Verification items for the finished model (mm, model axes). A direction names the side the tool comes from. Round coordinates to 2 decimals unless told otherwise and drop trailing zeros. Order: outer loops, then holes, each group sorted by start corner. A loop starts at its lowest first (then second) coordinate and runs counter-clockwise, first axis right, second up. Notation, with made-up numbers: (76, 79) -> (106, 79) arc R24 cw to (106, 116) -> close; hole circle Ø6 at (65.25, 62.25). An arc over 180 degrees is marked (long way). Return JSON: item names as keys, results as strings. Group by question number.
Item 1: Sectioned sample at A-A on x = 0. Record the cut outline in (y, z), plus the area to 3 significant figures.
Item 2: Depth check by flat-ended pin: pin 1 Ø9.5 at (x, y) = (-31.75, 54.99) entering from +Z; pin 2 Ø4 at (y, z) = (23, 4) entering from -X; pin 3 Ø5 at (y, z) = (31, 6) entering from -X. Enter the tip coordinate at first touch or a pass-through.
Item 3: Sectioned sample at B-B on z = -3.5. Record the cut outline in (x, y), plus the area to 3 significant figures.
Item 4: Access from +Z, -Z, +X, -X, +Y, -Y to the whole of each face (thin tool, end or side, straight path). Record for faces 4 (the cylindrical face through (-33.4, 51.83, 4.46)), 5 (the flat face through (62, 12.7, -3)).
Item 5: Scan lines: probe 1 along X at (y, z) = (31.75, 6.5); probe 2 along X at (y, z) = (67.5, 4.75); probe 3 along Z at (x, y) = (-49, 44). Record each from-to range of solid material in increasing order. Write a range as from..to.
Item 6: Draft check along X on faces 1 (the flat face through (-53, 2, 0)), 2 (the cylindrical face through (-58.29, 30.38, 4.46)), 3 (the flat face through (-1, 56, 12.7)). Enter one of: pulls with the +X half, pulls with the -X half, needs draft (parallel to the pull), parting line crosses it, or undercut.
Item 7: Sectioned sample at C-C on y = 42. Record the cut outline in (x, z), plus the area to 3 significant figures.
Item 8: Sectioned sample at D-D on z = 5. Record the cut outline in (x, y), plus the area to 3 significant figures.
```python
from build123d import *

# Parameters (mm, degrees)
F1_DEPTH       = 12.7
F3_DEPTH       = 6.35
F5_D           = 7.1374
F5_CSINK_D     = 13.4874
F5_CSINK_ANGLE = 82


with BuildPart() as f1:
    # F0 (on Top) → F1 (new body)
    with BuildSketch(Plane.XY):
        with BuildLine():
            Line((-76.2, 0), (-50.8, 0))
            ThreePointArc((-50.8, 0), (0, 50.8), (50.8, 0))
            Line((50.8, 0), (76.2, 0))
            ThreePointArc((76.2, 0), (0, 76.2), (-76.2, 0))
        make_face()
    extrude(amount=F1_DEPTH)

    # F2 (on face) → F3 (join)
    with BuildSketch(Plane(origin=(0, 0, 0), x_dir=(1, 0, 0), z_dir=(0, 0, -1))):
        with BuildLine():
            Line((-74.9170394667, -12.7), (-49.5170394667, -12.7))
            ThreePointArc((-49.5170394667, -12.7), (-49.581350313, -11.4235362865), (-49.7736315316, -10.1600002047))
            ThreePointArc((-49.7736315316, -10.1600002047), (-54.1848541289, -2.8626223667), (-62.2170394667, 0))
            ThreePointArc((-62.2170394667, 0), (-71.1972955878, -3.7197438789), (-74.9170394667, -12.7))
        make_face()
        with BuildLine():
            ThreePointArc((62.2170394667, 0), (54.1848541308, -2.8626223652), (49.7736315325, -10.1600001999))
            ThreePointArc((49.7736315325, -10.1600001999), (49.5813503133, -11.423536284), (49.5170394667, -12.7))
            Line((49.5170394667, -12.7), (74.9170394667, -12.7))
            ThreePointArc((74.9170394667, -12.7), (71.1972955878, -3.7197438789), (62.2170394667, 0))
        make_face()
    extrude(amount=F3_DEPTH)

    # F5 (through all)
    with Locations(Plane.XY.offset(12.7)):
        with Locations((-54.9926131403, 31.75), (-31.75, 54.9926131403), (0, 63.5), (31.75, 54.9926131403), (54.9926131403, 31.75)):
            CounterSinkHole(F5_D / 2, F5_CSINK_D / 2, counter_sink_angle=F5_CSINK_ANGLE)


solid = f1.part
```
Recorded:
{
 "1": {"outline": "(50.8, 0) -> (59.93, 0) -> (59.93, 9.05) -> (56.76, 12.7) -> (50.8, 12.7) -> close; (67.07, 0) -> (76.2, 0) -> (76.2, 12.7) -> (70.24, 12.7) -> (67.07, 9.05) -> close", "area": "220 mm²"},
 "2": {"pin 1": "z = 10.41", "pin 2": "x = -73.25", "pin 3": "x = -70.67"},
 "3": {"outline": "(-74.92, 12.7) arc R12.7 ccw to (-49.52, 12.7) -> close; (49.52, 12.7) arc R12.7 ccw to (74.92, 12.7) -> close", "area": "507 mm²"},
 "4": {"face 4": "+Z, -Z", "face 5": "-Z, +X, -X, +Y"},
 "5": {"probe 1": "-69.27..-58.56, -51.42..-39.66, 39.66..51.42, 58.56..69.27", "probe 2": "-35.36..35.36", "probe 3": "0..12.7"},
 "6": {"face 1": "undercut", "face 2": "undercut", "face 3": "needs draft"},
 "7": {"outline": "(-63.58, 0) -> (-28.58, 0) -> (-28.58, 12.7) -> (-63.58, 12.7) -> close; (28.58, 0) -> (63.58, 0) -> (63.58, 12.7) -> (28.58, 12.7) -> close", "area": "889 mm²"},
 "8": {"outline": "(-76.2, 0) -> (-50.8, 0) arc R50.8 cw to (50.8, 0) -> (76.2, 0) arc R76.2 ccw to start; hole circle Ø7.14 at (-54.99, 31.75); hole circle Ø7.14 at (-31.75, 54.99); hole circle Ø7.14 at (0, 63.5); hole circle Ø7.14 at (31.75, 54.99); hole circle Ø7.14 at (54.99, 31.75)", "area": "4,870 mm²"}
}
